Part model, mm, in its own coordinate system. A direction names the side the tool comes from. Round coordinates to 2 decimals unless told otherwise and drop trailing zeros. Write each loop counter-clockwise with the first axis right and the second up, starting at its lowest first coordinate (ties: lowest second). Pieces come first, ordered by that corner, then holes.
1) Saw through at B-B on y = 143. Write the cut outline in (x, z), and give its area (3 significant figures).
2) Saw through at A-A on y = 181. Write the cut outline in (x, z), and give its area (3 significant figures).
3) Drill centre lines: L1, parallel to Z at x = 1, y = 21; L2, parallel to Y at x = 20, z = -22.5; L3, parallel to X at y = 233, z = 10. Where is each one in solid material? Low to high.
4) Pull direction Y, two halves, no side cores. Call faces 3 (the cylindrical face through (-21, 42, -28)), 4 (the cylindrical face through (0.66, 227.888, -14.985)), 5 (the flat face through (-31.4, 85, 15.9)): +Y half, -Y half, draft (parallel to the pull), parting line (faces both ways), or undercut.
5) Flat gauge pins, fed straight in: pin 1 (12 mm diameter, centred on y = 266.5, z = -19, fed in from -X); pin 2 (4 mm diameter, centred on x = -14, y = 168, fed in from -Z); pin 3 (8 mm diameter, centred on x = -18, y = 130, fed in from -Z). Where does each tip first touch, or does it go through?
6) Which spindle directions (+Z, -Z, +X, -X, +Y, -Y) get a long thin tool onto all of the face, cutting with end or side? Do faces 1 (the cylindrical face through (-21, 183, -28)), 2 (the flat face through (0, 296, 0)). Say none if no direction does.
```python
from build123d import *

# Parameters (mm, degrees)
SKETCH2_R           = 35
BOSS_EXTRUDE1_DEPTH = 200
SKETCH3_R           = 15
BOSS_EXTRUDE2_DEPTH = 95
FILLET1_R           = 20
FILLET2_R           = 10
BOSS_EXTRUDE3_START = 1
SKETCH4_R           = 16
BOSS_EXTRUDE3_DEPTH = 60
BOSS_EXTRUDE4_START = -85
SKETCH5_R           = 35.5
BOSS_EXTRUDE4_DEPTH = 90


with BuildPart() as part:
    # Sketch2 → Boss-Extrude1 (new body)
    with BuildSketch(Plane(origin=(0, 0, 0), x_dir=(1, 0, 0), z_dir=(0, 1, 0))):
        with Locations(Location((0, 0, 0), (0, 0, 270))):
            Circle(SKETCH2_R)
    extrude(amount=BOSS_EXTRUDE1_DEPTH)

    # Sketch3 → Boss-Extrude2 (add)
    with BuildSketch(Plane(origin=(0, 200, 0), x_dir=(1, 0, 0), z_dir=(0, 1, 0))):
        with Locations(Location((0, 0, 0), (0, 0, 270))):
            Circle(SKETCH3_R)
    extrude(amount=BOSS_EXTRUDE2_DEPTH)

    # Fillet1
    fillet1_edges = [part.edges().sort_by_distance(p)[0] for p in [
        (0, 200, -15),
    ]]
    fillet(fillet1_edges, radius=FILLET1_R - 0.0001)  # a hair under: the kernel refuses the full size

    # Fillet2
    fillet2_edges = [part.edges().sort_by_distance(p)[0] for p in [
        (0, 200, -35),
    ]]
    fillet(fillet2_edges, radius=FILLET2_R)

    # Sketch4 → Boss-Extrude3 (add)
    with BuildSketch(Plane(origin=(0, 295, 0), x_dir=(1, 0, 0), z_dir=(0, 1, 0)).offset(BOSS_EXTRUDE3_START)):
        with Locations(Location((0, 0, 0), (0, 0, 270))):
            Circle(SKETCH4_R)
    extrude(amount=-BOSS_EXTRUDE3_DEPTH)

    # Sketch5 → Boss-Extrude4 (add)
    with BuildSketch(Plane.XZ.offset(BOSS_EXTRUDE4_START)):
        with Locations(Location((0, 0, 0), (0, 0, 270))):
            Circle(SKETCH5_R)
    extrude(amount=-BOSS_EXTRUDE4_DEPTH)


solid = part.part
```
Completed:
1. outline: circle Ø71 at (0, 0)
1. area: 3,960 mm2
2. outline: circle Ø70 at (0, 0)
2. area: 3,850 mm2
3. L1: z = -34.99 to 34.99
3. L2: y = 0 to 200.32
3. L3: x = -11.18 to 11.18
4. face 3: draft
4. face 4: undercut
4. face 5: -Y half
5. pin 1: stops at x = -9.33
5. pin 2: stops at z = -33.41
5. pin 3: stops at z = -32.62
6. face 1: +Y
6. face 2: +Z, -Z, +X, -X, +Y
